Job drawing, mm, ordinate dimensions from the low corner. One solid piece. Coordinates: 2 decimals unless noted, no trailing zeros. Loops run counter-clockwise (first coordinate to the right, second up) from the corner with the lowest first, then second, coordinate; pieces in that order, holes last. Notation, with made-up numbers: M -1.5,74 L 27.5,74 A11 ccw 27.5,83 Z; hole C -21,73 d2. An arc over 180 degrees is marked long. Answer as a JSON object with one key per item and string values. Group by question number.
1. Saw through at B-B on x = 28. Write the cut outline in (y, z).
2. Drill centre lines: L1, parallel to X at y = 8.5, z = 27.5; L2, parallel to X at y = 11.5, z = 1; L3, parallel to Z at x = 26, y = 5. Where is each one in solid material? Low to high.
3. Saw through at A-A on y = 4.75. Write the cut outline in (x, z), then the cut area to 3 significant figures.
4. Saw through at C-C on z = 2. Write the cut outline in (x, y).
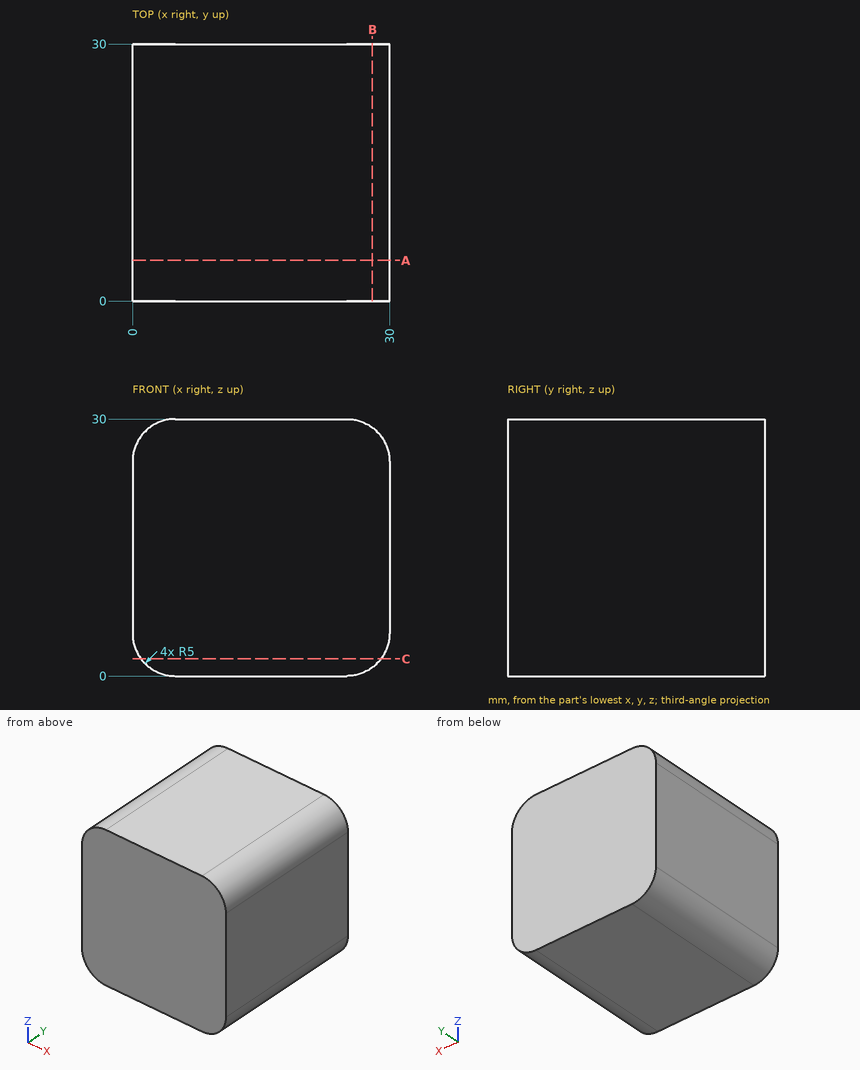
Outcome:
{
 "1": {"outline": "M 0,1 L 30,1 L 30,29 L 0,29 Z"},
 "2": {"L1": "x = 0.67 to 29.33", "L2": "x = 2 to 28", "L3": "z = 0.1 to 29.9"},
 "3": {"outline": "M 0,5 A5 ccw 5,0 L 25,0 A5 ccw 30,5 L 30,25 A5 ccw 25,30 L 5,30 A5 ccw 0,25 Z", "area": "879 mm²"},
 "4": {"outline": "M 1,0 L 29,0 L 29,30 L 1,30 Z"}
}
